Could you check a few things on this model? Use its own coordinates, in mm. Face numbers are marked on the shaded views. A direction names the side the tool comes from. Give positions to 0.01 mm unless a question says otherwise; leave off trailing zeros. Write each loop counter-clockwise with the first axis right and the second up, starting at its lowest first coordinate (ties: lowest second). Pieces come first, ordered by that corner, then holes. Notation, with made-up numbers: (53, 15.25) -> (99, 15.25) arc R22 ccw to (99, 30.25) -> close; hole circle Ø10 at (75, 0.5). An arc over 180 degrees is marked (long way). Write item = value, one per line. Start each with the question number.
```python
from build123d import *

# Parameters (mm, degrees)
BOSS_EXTRUDE1_DEPTH = 30
CUT_EXTRUDE1_START  = -1.5
CUT_EXTRUDE1_DEPTH  = 27
CUT_EXTRUDE2_DEPTH  = 42.833001327
CUT_EXTRUDE3_DEPTH  = 50.244289009
SKETCH8_W           = 30
SKETCH8_H           = 30
SKETCH8_W_2         = 29
SKETCH8_H_2         = 29
CUT_EXTRUDE5_DEPTH  = 1
CUT_EXTRUDE9_START  = -31
SKETCH9_W           = 30
SKETCH9_H           = 30
SKETCH9_W_2         = 29
SKETCH9_H_2         = 29
CUT_EXTRUDE9_DEPTH  = 0.5


with BuildPart() as part:
    # Sketch1 → Boss-Extrude1 (new body)
    with BuildSketch(Plane.XY):
        with BuildLine():
            Line((-15, -25), (15, -25))
            Line((15, -25), (15, 22))
            ThreePointArc((15, 22), (14.121320344, 24.121320344), (12, 25))
            Line((12, 25), (-12, 25))
            ThreePointArc((-12, 25), (-14.121320344, 24.121320344), (-15, 22))
            Line((-15, 22), (-15, -25))
        make_face()
    extrude(amount=-BOSS_EXTRUDE1_DEPTH)

    # Sketch2 → Cut-Extrude1 (cut)
    with BuildSketch(Plane.XY.offset(CUT_EXTRUDE1_START)):
        with BuildLine():
            Line((-13, 22), (-13, -23))
            Line((-13, -23), (13, -23))
            Line((13, -23), (13, 22))
            ThreePointArc((13, 22), (12.707106781, 22.707106781), (12, 23))
            Line((12, 23), (-12, 23))
            ThreePointArc((-12, 23), (-12.707106781, 22.707106781), (-13, 22))
        make_face()
    extrude(amount=-CUT_EXTRUDE1_DEPTH, mode=Mode.SUBTRACT)

    # Sketch4 → Cut-Extrude2 (cut, through all)
    with BuildSketch(Plane.XY):
        with BuildLine():
            ThreePointArc((-11, 20), (-10.414213562, 21.414213562), (-9, 22))
            Line((-9, 22), (9, 22))
            ThreePointArc((9, 22), (10.414213562, 21.414213562), (11, 20))
            Line((11, 20), (11, 11.5))
            ThreePointArc((11, 11.5), (10.414213562, 10.085786438), (9, 9.5))
            Line((9, 9.5), (-9, 9.5))
            ThreePointArc((-9, 9.5), (-10.414213562, 10.085786438), (-11, 11.5))
            Line((-11, 11.5), (-11, 20))
        make_face()
    extrude(amount=-CUT_EXTRUDE2_DEPTH, mode=Mode.SUBTRACT)

    # Sketch5 → Cut-Extrude3 (cut, through all)
    with BuildSketch(Plane(origin=(15, 0, 0), x_dir=(0, 0, -1), z_dir=(1, 0, 0))):
        with BuildLine():
            Line((6, 22), (24, 22))
            ThreePointArc((24, 22), (25.414213562, 21.414213562), (26, 20))
            Line((26, 20), (26, 11.5))
            ThreePointArc((26, 11.5), (25.414213562, 10.085786438), (24, 9.5))
            Line((24, 9.5), (6, 9.5))
            ThreePointArc((6, 9.5), (4.585786438, 10.085786438), (4, 11.5))
            Line((4, 11.5), (4, 20))
            ThreePointArc((4, 20), (4.585786438, 21.414213562), (6, 22))
        make_face()
    extrude(amount=-CUT_EXTRUDE3_DEPTH, mode=Mode.SUBTRACT)

    # Sketch8 → Cut-Extrude5 (cut)
    with BuildSketch(Plane.XZ.offset(25)):
        with Locations((0, -15)):
            Rectangle(SKETCH8_W, SKETCH8_H)
        with Locations((0, -15)):
            Rectangle(SKETCH8_W_2, SKETCH8_H_2, mode=Mode.SUBTRACT)
    extrude(amount=-CUT_EXTRUDE5_DEPTH, mode=Mode.SUBTRACT)

    # Sketch9 → Cut-Extrude9 (cut)
    with BuildSketch(Plane.XZ.offset(24).offset(CUT_EXTRUDE9_START)):
        with Locations((0, -15)):
            Rectangle(SKETCH9_W, SKETCH9_H)
        with Locations((0, -15)):
            Rectangle(SKETCH9_W_2, SKETCH9_H_2, mode=Mode.SUBTRACT)
    extrude(amount=CUT_EXTRUDE9_DEPTH, mode=Mode.SUBTRACT)


solid = part.part
```
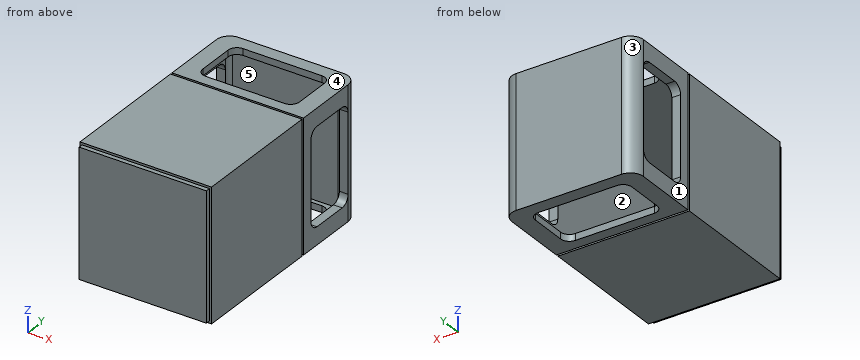
(1) Imagine slicing it at C-C (x = -2.5). Please give me the cut outline in (y, z).
(2) On a 3-axis mill with a long thin cutter (end or side, diameter ignored), from which of +Z, -Z, +X, -X, +Y, -Y can I reach the whole of each face in a straight line? I mean the marked faces 4 and 5. Say none if no direction works.
(3) We'd pull the mould along Y, two halves only. Please class the marked faces 1, 2 and 3: released by +Y, released by -Y, zero draft, split by the parting line, or undercut.
(4) I'm going to push flat-ended pins straight in: pin 1 (0.8 mm diameter, centred on x = -7, y = -24.5, fed in from +Z); pin 2 (1 mm diameter, centred on x = -14, z = -12, fed in from +Y); pin 3 (0.8 mm diameter, centred on y = -24.5, z = -13, fed in from -X). Where does each tip first touch, or does it pass through?
(5) Imagine slicing it at A-A (y = 0). Please give me the cut outline in (x, z), then the cut area to 3 significant figures.
(6) If I drill on line 1 along Z through (x, y) = (7, -1); line 2 along X through (y, z) = (5, -17); line 3 along Y through (x, z) = (-7.5, -17.75), over which ranges is the centre line in solid material (lowest first)? Write a range as from..to.
(7) Imagine slicing it at B-B (z = -12.25). Please give me the cut outline in (x, y).
Answers below:
q1.outline = (-25, -29.5) -> (-24, -29.5) -> (-24, -30) -> (6.5, -30) -> (6.5, -29.5) -> (7, -29.5) -> (7, -30) -> (9.5, -30) -> (9.5, -28.5) -> (-23, -28.5) -> (-23, -1.5) -> (9.5, -1.5) -> (9.5, 0) -> (7, 0) -> (7, -0.5) -> (6.5, -0.5) -> (6.5, 0) -> (-24, 0) -> (-24, -0.5) -> (-25, -0.5) -> close; (22, -30) -> (25, -30) -> (25, 0) -> (22, 0) -> (22, -1.5) -> (23, -1.5) -> (23, -28.5) -> (22, -28.5) -> close
q2.face_4 = +Z, +X, -X, +Y, -Y
q2.face_5 = none
q3.face_1 = zero draft
q3.face_2 = undercut
q3.face_3 = released by +Y
q4.pin_1 = -0.5
q4.pin_2 = 24.6
q4.pin_3 = -14.5
q5.outline = (-15, -30) -> (15, -30) -> (15, 0) -> (-15, 0) -> close; hole (-13, -28.5) -> (13, -28.5) -> (13, -1.5) -> (-13, -1.5) -> close
q5.area = 198 mm^2
q6.line_1 = -30..-28.5, -1.5..0
q6.line_2 = -15..-13, 13..15
q6.line_3 = -25..-23, 23..25
q7.outline = (-15, -24) -> (-14.5, -24) -> (-14.5, -25) -> (14.5, -25) -> (14.5, -24) -> (15, -24) -> (15, 6.5) -> (14.5, 6.5) -> (14.5, 7) -> (15, 7) -> (15, 9.5) -> (13, 9.5) -> (13, -23) -> (-13, -23) -> (-13, 9.5) -> (-15, 9.5) -> (-15, 7) -> (-14.5, 7) -> (-14.5, 6.5) -> (-15, 6.5) -> close; (-15, 22) -> (-13, 22) arc R1 cw to (-12, 23) -> (12, 23) arc R1 cw to (13, 22) -> (15, 22) arc R3 ccw to (12, 25) -> (-12, 25) arc R3 ccw to start
